Part model, mm, in its own coordinate system. Give positions to 0.01 mm unless a question says otherwise; leave off trailing zeros. Order: outer loops, then holes, each group sorted by start corner. A loop starts at its lowest first (then second) coordinate and runs counter-clockwise, first axis right, second up.
1. Slice it at B-B on y = -28. List the corners of the cut face in (x, z), and give its area (3 significant figures).
2. Probe line 1 (Y direction, x = 77, z = 2.3); line 2 (X direction, y = -14, z = 2.85); line 3 (Y direction, x = 10, z = 0.4). List the from-to ranges inside material, lowest first.
3. Slice it at A-A on x = 35.5. List the corners of the cut face in (y, z), and give its area (3 significant figures).
4. Slice it at C-C on z = 1.25. List the corners of the cut face in (x, y), and give its area (3 significant figures).
from build123d import *

# Parameters (mm, degrees)
SKETCH_1_R          = 1.6
EXTRUDE_1_DEPTH     = 3
SKETCH_3_W          = 57.604070615
SKETCH_3_H          = 38.574154429
CUT_EXTRUDE_1_DEPTH = 10


with BuildPart() as part:
    # 草图1 → 凸台-拉伸1 (new body)
    with BuildSketch(Plane.XY):
        with BuildLine():
            Line((0, -52), (77, -52))
            ThreePointArc((77, -52), (79.121320344, -51.121320344), (80, -49))
            Line((80, -49), (80, 0))
            ThreePointArc((80, 0), (79.121320344, 2.121320344), (77, 3))
            Line((77, 3), (0, 3))
            ThreePointArc((0, 3), (-2.121320344, 2.121320344), (-3, 0))
            Line((-3, 0), (-3, -49))
            ThreePointArc((-3, -49), (-2.121320344, -51.121320344), (0, -52))
        make_face()
        Circle(SKETCH_1_R, mode=Mode.SUBTRACT)
        with Locations((77, 0)):
            Circle(SKETCH_1_R, mode=Mode.SUBTRACT)
        with Locations((0, -49)):
            Circle(SKETCH_1_R, mode=Mode.SUBTRACT)
        with Locations((77, -49)):
            Circle(SKETCH_1_R, mode=Mode.SUBTRACT)
        with BuildLine():
            Line((16.5, -41.5), (60.5, -41.5))
            ThreePointArc((60.5, -41.5), (62.621320344, -40.621320344), (63.5, -38.5))
            Line((63.5, -38.5), (63.5, -10.5))
            ThreePointArc((63.5, -10.5), (62.621320344, -8.378679656), (60.5, -7.5))
            Line((60.5, -7.5), (16.5, -7.5))
            ThreePointArc((16.5, -7.5), (14.378679656, -8.378679656), (13.5, -10.5))
            Line((13.5, -10.5), (13.5, -38.5))
            ThreePointArc((13.5, -38.5), (14.378679656, -40.621320344), (16.5, -41.5))
        make_face(mode=Mode.SUBTRACT)
    extrude(amount=EXTRUDE_1_DEPTH)

    # 草图3 → 切除-拉伸1 (cut)
    with BuildSketch(Plane.XY.offset(3)):
        with Locations((38.662365372, -24.543784479)):
            Rectangle(SKETCH_3_W, SKETCH_3_H)
    extrude(amount=-CUT_EXTRUDE_1_DEPTH, mode=Mode.SUBTRACT)


solid = part.part
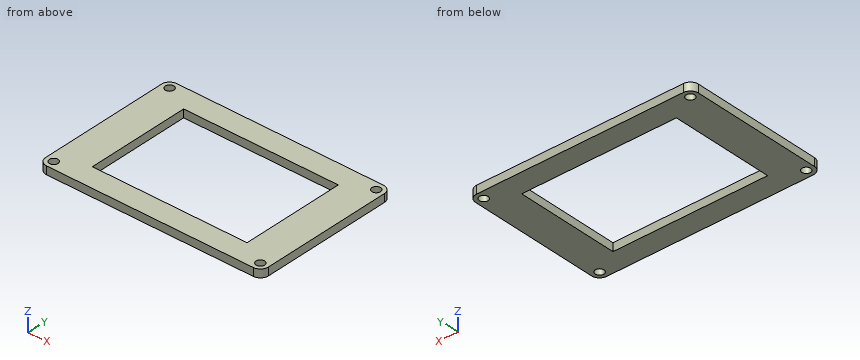
Data:
1. outline: (-3, 0) - (9.86, 0) - (9.86, 3) - (-3, 3) - close; (67.46, 0) - (80, 0) - (80, 3) - (67.46, 3) - close
1. area: 76.2 mm2
2. line 1: y = -52 to -50.6, -47.4 to -1.6, 1.6 to 3
2. line 2: x = -3 to 9.86, 67.46 to 80
2. line 3: y = -52 to -43.83, -5.26 to 3
3. outline: (-52, 0) - (-43.83, 0) - (-43.83, 3) - (-52, 3) - close; (-5.26, 0) - (3, 0) - (3, 3) - (-5.26, 3) - close
3. area: 49.3 mm2
4. outline: (-3, -49) arc R3 ccw to (0, -52) - (77, -52) arc R3 ccw to (80, -49) - (80, 0) arc R3 ccw to (77, 3) - (0, 3) arc R3 ccw to (-3, 0) - close; hole circle Ø3.2 at (0, -49); hole circle Ø3.2 at (0, 0); hole (9.86, -43.83) - (67.46, -43.83) - (67.46, -5.26) - (9.86, -5.26) - close; hole circle Ø3.2 at (77, -49); hole circle Ø3.2 at (77, 0)
4. area: 2,300 mm2
